```python
from build123d import *

# Parameters (mm, degrees)
SKETCH_1_R          = 1.3
SKETCH_1_R_2        = 6.5
EXTRUDE_1_DEPTH     = 4
CUT_EXTRUDE_1_DEPTH = 2
CUT_EXTRUDE_2_DEPTH = 10
EXTRUDE_START       = -4
EXTRUDE_2_DEPTH     = 4
FILLET_1_R          = 5
SKETCH_5_R          = 1.65
CUT_EXTRUDE_3_DEPTH = 10
SKETCH_6_R          = 3.5
SKETCH_6_R_2        = 2.25
CUT_EXTRUDE_4_DEPTH = 2


with BuildPart() as part:
    # 草图1 → 凸台-拉伸1 (new body)
    with BuildSketch(Plane.XY):
        with BuildLine():
            Line((8.553461717, -18.071837398), (16.553461717, -18.071837398))
            Line((16.553461717, -18.071837398), (22.424329469, 1.203351624))
            ThreePointArc((22.424329469, 1.203351624), (19.185042818, 15.288156683), (5.383718421, 19.577463907))
            Line((5.383718421, 19.577463907), (-21.197136513, 13.622789192))
            Line((-21.197136513, 13.622789192), (-12.744771278, -4.503366549))
            ThreePointArc((-12.744771278, -4.503366549), (-4.073079079, -14.391536375), (8.553461717, -18.071837398))
        make_face()
        with Locations((16.780703053, 10.178162602)):
            Circle(SKETCH_1_R, mode=Mode.SUBTRACT)
        with Locations((8.553461717, -4.071837398)):
            Circle(SKETCH_1_R, mode=Mode.SUBTRACT)
        with Locations((8.553461717, 5.428162602)):
            Circle(SKETCH_1_R_2, mode=Mode.SUBTRACT)
        with Locations((0.326220381, 10.178162602)):
            Circle(SKETCH_1_R, mode=Mode.SUBTRACT)
    extrude(amount=EXTRUDE_1_DEPTH)

    # 草图2 → 切除-拉伸1 (cut)
    with BuildSketch(Plane.XY.offset(4)):
        with BuildLine():
            Line((-20.74398262, 13.834098323), (-26.791770356, 13.834098323))
            Line((-26.791770356, 13.834098323), (-7.810487919, -16.678792008))
            Line((-7.810487919, -16.678792008), (17.290442954, -20.516537637))
            Line((17.290442954, -20.516537637), (21.405478984, -18.597664823))
            Line((21.405478984, -18.597664823), (16.553461717, -17.571837398))
            Line((16.553461717, -17.571837398), (8.553461717, -17.571837398))
            ThreePointArc((8.553461717, -17.571837398), (-3.804429275, -13.969840652), (-12.291617385, -4.292057418))
            Line((-12.291617385, -4.292057418), (-20.74398262, 13.834098323))
        make_face()
    extrude(amount=-CUT_EXTRUDE_1_DEPTH, mode=Mode.SUBTRACT)

    # 草图3 → 切除-拉伸2 (cut)
    with BuildSketch(Plane.XY.offset(4)):
        with BuildLine():
            Line((16.553461717, -18.071837398), (16.696538979, -17.602087204))
            Line((16.696538979, -17.602087204), (16.553461717, -17.571837398))
            Line((16.553461717, -17.571837398), (8.553461717, -17.571837398))
            ThreePointArc((8.553461717, -17.571837398), (-3.804429275, -13.969840652), (-12.291617385, -4.292057418))
            Line((-12.291617385, -4.292057418), (-20.697627647, 13.734689762))
            Line((-20.697627647, 13.734689762), (-21.197136513, 13.622789192))
            Line((-21.197136513, 13.622789192), (-12.744771278, -4.503366549))
            ThreePointArc((-12.744771278, -4.503366549), (-4.073079079, -14.391536375), (8.553461717, -18.071837398))
            Line((8.553461717, -18.071837398), (16.553461717, -18.071837398))
        make_face()
    extrude(amount=-CUT_EXTRUDE_2_DEPTH, mode=Mode.SUBTRACT)

    # 草图4 → 凸台-拉伸2 (add)
    with BuildSketch(Plane.XY.offset(4).offset(EXTRUDE_START)):
        with BuildLine():
            Line((5.383718421, 19.577463907), (29.678441091, 25.019996556))
            Line((29.678441091, 25.019996556), (22.424329469, 1.203351624))
            ThreePointArc((22.424329469, 1.203351624), (19.185042818, 15.288156683), (5.383718421, 19.577463907))
        make_face()
    extrude(amount=EXTRUDE_2_DEPTH)

    # 圆角1
    fillet_1_edges = [part.edges().sort_by_distance(p)[0] for p in [
        (29.678441091, 25.019996556, 2),
    ]]
    fillet(fillet_1_edges, radius=FILLET_1_R)

    # 草图5 → 切除-拉伸3 (cut)
    with BuildSketch(Plane.XY.offset(4)):
        with Locations((22.393965445, 18.264191744)):
            Circle(SKETCH_5_R)
        with Locations((-9.483117468, 10.99637586)):
            Circle(SKETCH_5_R)
        with Locations((12.749537174, -12.976079799)):
            Circle(SKETCH_5_R)
    extrude(amount=-CUT_EXTRUDE_3_DEPTH, mode=Mode.SUBTRACT)

    # 草图6 → 切除-拉伸4 (cut)
    with BuildSketch(Plane.XY.offset(4)):
        with Locations((22.393965445, 18.264191744)):
            Circle(SKETCH_6_R)
        with Locations((-9.483117468, 10.99637586)):
            Circle(SKETCH_6_R)
        with Locations((12.749537174, -12.976079799)):
            Circle(SKETCH_6_R)
        with Locations((8.553461717, -4.071837398)):
            Circle(SKETCH_6_R_2)
        with Locations((16.780703053, 10.178162602)):
            Circle(SKETCH_6_R_2)
        with Locations((0.326220381, 10.178162602)):
            Circle(SKETCH_6_R_2)
    extrude(amount=-CUT_EXTRUDE_4_DEPTH, mode=Mode.SUBTRACT)


solid = part.part
```
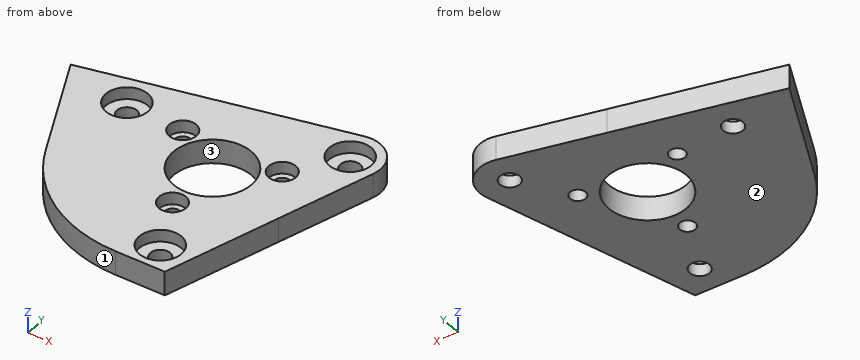
Could you check a few things on this model? Use its own coordinates, in mm. Face numbers are marked on the shaded views. Coordinates: 2 decimals unless noted, no trailing zeros. Write each loop counter-clockwise with the first axis right and the second up, starting at its lowest first coordinate (ties: lowest second). Pieces come first, ordered by that corner, then holes. Notation, with made-up numbers: (-39.5, 25) -> (19.5, 25) arc R17 ccw to (19.5, 47) -> close; hole circle Ø8 at (43, 75). An arc over 180 degrees is marked (long way). Write item = value, one per line. Start each with the question number.
(1) I want a section at B-B (x = 23). Please give me the cut outline in (y, z), plus the area to 3 significant figures.
(2) I want a section at C-C (z = 3.4). Please give me the cut outline in (x, y).
(3) Will these pins go through, and if not, where does the flat tip stop? pin 1 (6 mm diameter, centred on x = 16.78, y = 10.18, fed in from +Z); pin 2 (4.5 mm diameter, centred on x = 22.39, y = 18.26, fed in from +Z); pin 3 (1.5 mm diameter, centred on x = -11, z = 2, fed in from -Y); pin 4 (2 mm diameter, centred on x = -4.5, z = 2, fed in from +Y).
(4) We'd pull the mould along Y, two halves only. Please class the marked faces 1, 2 and 3: released by +Y, released by -Y, zero draft, split by the parting line, or undercut.
(5) I want a section at D-D (y = 4). Please give me the cut outline in (x, z).
(6) I want a section at A-A (y = -12). Please give me the cut outline in (x, z).
(7) I need wall thicknesses on line 1 (X direction, y = 9, z = 2.2); line 2 (Y direction, x = 7.5, z = 3.25); line 3 (Y direction, x = 14.5, z = 3.45). Which ranges of each line are inside material? Lowest first, please. Write a range as [from, to].
Result set:
q1.outline = (3.09, 0) -> (16.73, 0) -> (16.73, 2) -> (14.82, 2) -> (14.82, 4) -> (3.09, 4) -> close; (19.8, 0) -> (23.23, 0) -> (23.23, 4) -> (21.71, 4) -> (21.71, 2) -> (19.8, 2) -> close
q1.area = 60.6 mm2
q2.outline = (-20.7, 13.73) -> (-12.29, -4.29) arc R23 ccw to (8.55, -17.57) -> (16.55, -17.57) -> (16.7, -17.6) -> (27.18, 16.81) arc R5 ccw to (21.3, 23.14) -> close; hole circle Ø7 at (-9.48, 11); hole circle Ø4.5 at (0.33, 10.18); hole circle Ø13 at (8.55, 5.43); hole circle Ø4.5 at (8.55, -4.07); hole circle Ø7 at (12.75, -12.98); hole circle Ø4.5 at (16.78, 10.18); hole circle Ø7 at (22.39, 18.26)
q3.pin_1 = 4
q3.pin_2 = 2
q3.pin_3 = -7.82
q3.pin_4 = 17.59
q4.face_1 = released by -Y
q4.face_2 = zero draft
q4.face_3 = undercut
q5.outline = (-16.16, 0) -> (2.21, 0) -> (2.21, 4) -> (-16.16, 4) -> close; (14.89, 0) -> (23.28, 0) -> (23.28, 4) -> (14.89, 4) -> close
q6.outline = (-6.46, 0) -> (11.42, 0) -> (11.42, 2) -> (9.39, 2) -> (9.39, 4) -> (-6.46, 4) -> close; (14.08, 0) -> (18.4, 0) -> (18.4, 4) -> (16.11, 4) -> (16.11, 2) -> (14.08, 2) -> close
q7.line_1 = [-18.49, -12.36], [-6.61, -1.59], [2.24, 3.12], [13.98, 14.86], [18.7, 24.8]
q7.line_2 = [-17.55, -6.06], [-2.08, -0.99], [11.84, 20.05]
q7.line_3 = [-17.57, -16.01], [-9.95, 2.8], [8.05, 21.62]
